Part model, mm, in its own coordinate system. Face numbers are marked on the shaded views. A direction names the side the tool comes from. Give positions to 0.01 mm unless a question says otherwise; leave off trailing zeros. Loops run counter-clockwise (first coordinate to the right, second up) from the corner with the lowest first, then second, coordinate; pieces in that order, holes last. Notation, with made-up numbers: M 58,-19 L 90,-19 A15 cw 90,1 Z; hole C 49.5,22.5 d7. An arc over 180 degrees is marked long. Answer in a Markdown table with one row per item.
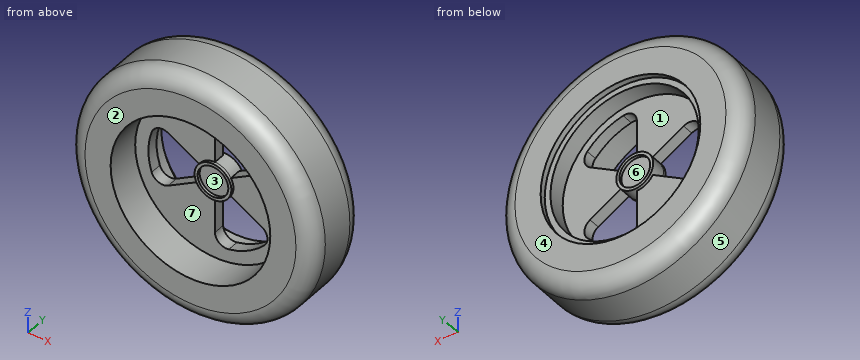
Autodesk Fusion 360 part; units mm, degrees
sketch "Sketch1" plane through (0, 0, 0) normal (0, 1, 0) x (1, 0, 0)
  circle A0 centre (0, 0) radius 21.5
  circle A1 centre (0, 0) radius 14
  circle A2 centre (0, 0) radius 13
  dimension "d1" = 43
  dimension "d2" = 28
  dimension "d3" = 26
extrude "Extrude1" add sketch "Sketch1" along normal mid plane 12 contours A0
extrude "Extrude2" add sketch "Sketch1" along normal blind 5 contours A1
extrude "Extrude3" add sketch "Sketch1" along normal blind 2 contours A2
fillet "Fillet1" radius 3 2 edges at (-20.045, 6, 7.7747) (-20.045, -6, -7.7747)
sketch "Sketch2" plane through (0, 2, 0) normal (0, 1, 0) x (-1, 0, 0)
  circle A0 centre (0, 0) radius 13
  line L0 (0, 0) -> (0, -13)
  line L1 (0, 0) -> (-11.253, 6.5092)
  line L2 (0, 0) -> (11.253, 6.5092)
  line L3 (0, 0) -> (-11.253, -6.5092)
  line L4 (0, 0) -> (0, 13)
  line L5 (11.253, -6.5092) -> (-11.253, 6.5092)
  circle A1 centre (0, 0) radius 11.6863
extrude "Extrude4" cut sketch "Sketch2" against normal blind 17 contours L2 L5 A1 | L1 L4 L5 A1 | L0 L3 A1
fillet "Fillet2" radius 2 6 edges at (0, 1, -11.6863) (10.1158, 1, 5.8514) (0, 1, 11.6863) (-10.1158, 1, 5.8514) (10.1158, 1, -5.8514) (-10.1158, 1, -5.8514)
sketch "Sketch3" plane through (0, 2, 0) normal (0, 1, 0) x (-1, 0, 0)
  arc A0 (11.106, -3.6366) -> (11.106, 3.6366) centre (0, 0) ccw
  arc A1 (8.2039, -4.7455) -> (11.106, -3.6366) centre (9.2053, -3.0142) ccw
  line L0 (8.2039, -4.7455) -> (0, 0)
  line L1 (0, 0) -> (0, -9.4775)
  arc A2 (-2.413, -11.4344) -> (0, -9.4775) centre (-2, -9.4775) ccw
  arc A3 (-8.6897, -7.814) -> (-2.413, -11.4344) centre (0, 0) ccw
  arc A4 (-8.2039, -4.7455) -> (-8.6897, -7.814) centre (-7.2025, -6.4767) ccw
  line L2 (-8.2039, -4.7455) -> (0, 0)
  line L3 (0, 0) -> (-8.2039, 4.7455)
  arc A5 (-8.6897, 7.814) -> (-8.2039, 4.7455) centre (-7.2025, 6.4767) ccw
  arc A6 (-2.413, 11.4344) -> (-8.6897, 7.814) centre (0, 0) ccw
  arc A7 (0, 9.4775) -> (-2.413, 11.4344) centre (-2, 9.4775) ccw
  line L4 (0, 9.4775) -> (0, 0)
  line L5 (0, 0) -> (8.2039, 4.7455)
  arc A8 (11.106, 3.6366) -> (8.2039, 4.7455) centre (9.2053, 3.0142) ccw
  circle A9 centre (0, 0) radius 13
  circle A10 centre (0, 0) radius 3.2281
  circle A11 centre (0, 0) radius 2.7011
extrude "Extrude5" add sketch "Sketch3" against normal blind 2 contours L0 L1 A10 A11 | L0 L5 A10 A11 | L4 L5 A10 A11 | L0 L1 A11 | L0 L5 A11 | L1 L2 A10 A11 | L4 L5 A11 | L3 L4 A10 A11 | L1 L2 A11 | L2 L3 A11 | L3 L4 A11 | L2 L3 A10 A11
sketch "Sketch4" plane through (0, 2, 0) normal (0, 1, 0) x (-1, 0, 0)
  line L0 (0, -3.2281) -> (0, -9.4775)
  arc A0 (-2.413, -11.4344) -> (0, -9.4775) centre (-2, -9.4775) ccw
  arc A1 (-8.6897, -7.814) -> (-2.413, -11.4344) centre (0, 0) ccw
  arc A2 (-8.2039, -4.7455) -> (-8.6897, -7.814) centre (-7.2025, -6.4767) ccw
  line L1 (-8.2039, -4.7455) -> (-2.7943, -1.6163)
  arc A3 (-2.7943, -1.6163) -> (0, -3.2281) centre (0, 0) ccw
  line L2 (-2.7943, 1.6163) -> (-8.2039, 4.7455)
  arc A4 (-8.6897, 7.814) -> (-8.2039, 4.7455) centre (-7.2025, 6.4767) ccw
  arc A5 (-2.413, 11.4344) -> (-8.6897, 7.814) centre (0, 0) ccw
  arc A6 (0, 9.4775) -> (-2.413, 11.4344) centre (-2, 9.4775) ccw
  line L3 (0, 9.4775) -> (0, 3.2281)
  arc A7 (0, 3.2281) -> (-2.7943, 1.6163) centre (0, 0) ccw
  arc A8 (2.7943, -1.6163) -> (2.7943, 1.6163) centre (0, 0) ccw
  line L4 (2.7943, 1.6163) -> (8.2039, 4.7455)
  arc A9 (11.106, 3.6366) -> (8.2039, 4.7455) centre (9.2053, 3.0142) ccw
  arc A10 (11.106, -3.6366) -> (11.106, 3.6366) centre (0, 0) ccw
  arc A11 (8.2039, -4.7455) -> (11.106, -3.6366) centre (9.2053, -3.0142) ccw
  line L5 (8.2039, -4.7455) -> (2.7943, -1.6163)
  circle A12 centre (0, 0) radius 13
  circle A13 centre (0, 0) radius 3.25
  circle A14 centre (0, 0) radius 2.7033
  circle A15 centre (0, 0) radius 2.7011
  circle A16 centre (0, 0) radius 3.2281
  circle A17 centre (0, 0) radius 3.25
  dimension "d18" = 6.5
extrude "Extrude6" add sketch "Sketch3" along normal blind 0.5 contours L0 L1 A10 A11 | L0 L5 A10 A11 | L4 L5 A10 A11 | L1 L2 A10 A11 | L3 L4 A10 A11 | L2 L3 A10 A11
sketch "Sketch5" plane through (0, 0, 0) normal (0, 1, 0) x (1, 0, 0)
  circle A0 centre (0, 0) radius 3.2294
  circle A1 centre (0, 0) radius 2.6936
extrude "Extrude7" add sketch "Sketch5" against normal blind 0.5
(1) Pin check, flat tips, straight feed: pin 1 Ø1.6 at (y, z) = (1, -5.5) entering from +X; pin 2 Ø6 at (x, y) = (-8.5, -2) entering from +Z; pin 3 Ø1.5 at (y, z) = (-4, 12.5) entering from -X (3 decimals). Stop position of each tip, or through.
Recorded:
| item | result |
|---|---|
| pin 1 | stops at x = 20.98 |
| pin 2 | stops at z = 20.78 |
| pin 3 | stops at x = -17.865 |
(2) Saw through at A-A (y = -5). Write the cut outline in (x, z).
Recorded:
| item | result |
|---|---|
| outline | C 0,0 d41.47; hole C 0,0 d28 |
(3) Saw through at B-B (x = 5.5). Give the number of separate pieces and of enclosed holes in the cut face, plus the area to 3 significant figures.
Recorded:
| item | result |
|---|---|
| separate pieces | 3 |
| enclosed holes | 0 |
| area | 211 mm^2 |
(4) Which spindle directions (+Z, -Z, +X, -X, +Y, -Y) get a long thin tool onto all of the face, cutting with end or side? Do the marked faces 1, 2 and 3. Say none if no direction does.
Recorded:
| item | result |
|---|---|
| face 1 | +Y |
| face 2 | +Z, -Z, +X, -X, -Y |
| face 3 | -Y |
(5) Drill centre lines: line 1 along Z through (x, y) = (0, -0.2); line 2 along X through (y, z) = (2.15, 0). Where is each one in solid material? Low to high.
Recorded:
| item | result |
|---|---|
| line 1 | z = -21.5 to -14, -3.23 to -2.69, 2.69 to 3.23, 14 to 21.5 |
| line 2 | x = -21.5 to -13, -3.23 to -2.7, 2.7 to 3.23, 13 to 21.5 |
(6) Pull direction Z, two halves, no side cores. Call the marked faces 4, 5, 6 and 7: +Z half, -Z half, draft (parallel to the pull), parting line (faces both ways), or undercut.
Recorded:
| item | result |
|---|---|
| face 4 | draft |
| face 5 | parting line |
| face 6 | undercut |
| face 7 | undercut |
